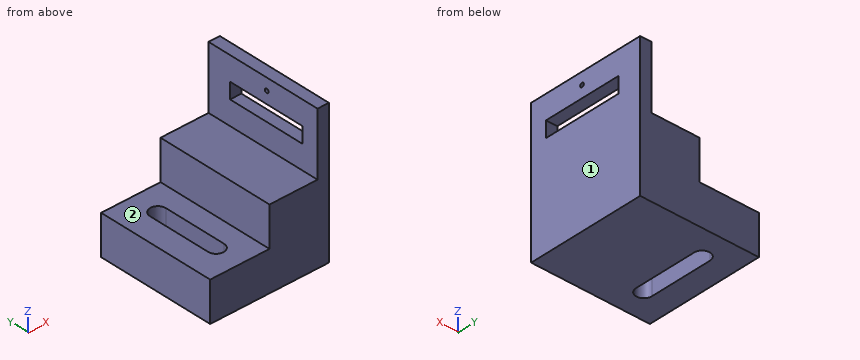
```python
from build123d import *

# Parameters (mm, degrees)
F1_DEPTH = 150
F3_DEPTH = 50.001
F4_W     = 100
F4_H     = 20
F4_R     = 2.5
F5_DEPTH = 14.313931


with BuildPart() as f1:
    # F0 (on Front) → F1 (new body)
    with BuildSketch(Plane.XZ):
        Polygon((-75, -90), (75, -90), (75, 90), (60.687069, 90), (60.687069, 10), (0, 10), (0, -40), (-75, -40), align=None)
    extrude(amount=F1_DEPTH)

    # F2 (on face) → F3 (cut, through all)
    with BuildSketch(Plane.XY.offset(-40)):
        with BuildLine():
            ThreePointArc((-45.374333, -35), (-35.374333, -45), (-25.374333, -35))
            ThreePointArc((-25.374333, -35), (-35.374333, -25), (-45.374333, -35))
        make_face()
        with BuildLine():
            Line((-25.374333, -115), (-25.374333, -35))
            ThreePointArc((-25.374333, -35), (-35.374333, -45), (-45.374333, -35))
            Line((-45.374333, -35), (-45.374333, -115))
            ThreePointArc((-45.374333, -115), (-35.374333, -105), (-25.374333, -115))
        make_face()
        with BuildLine():
            ThreePointArc((-45.374333, -115), (-35.374333, -125), (-25.374333, -115))
            ThreePointArc((-25.374333, -115), (-35.374333, -105), (-45.374333, -115))
        make_face()
    extrude(amount=-F3_DEPTH, mode=Mode.SUBTRACT)

    # F4 (on face) → F5 (cut, through all)
    with BuildSketch(Plane(origin=(60.687069, 0, 0), x_dir=(0, -1, 0), z_dir=(-1, 0, 0))):
        with Locations((79.612304, 50)):
            Rectangle(F4_W, F4_H)
        with Locations((80.003977, 75)):
            Circle(F4_R)
    extrude(amount=-F5_DEPTH, mode=Mode.SUBTRACT)


solid = f1.part
```
The listing builds one solid part. Answer for the finished solid, in the listing's coordinates (mm). Face numbers are marked on the shaded views. A direction names the side the tool comes from. Coordinates: 2 decimals unless noted, no trailing zeros. Write each loop counter-clockwise with the first axis right and the second up, starting at its lowest first coordinate (ties: lowest second). Pieces come first, ordered by that corner, then holes. Notation, with made-up numbers: M -26,32 L 18,32 A15 cw 18,59 Z; hole C 69,-8.75 d6. An arc over 180 degrees is marked long. Use a Markdown table: item, result. Add a question column.
1. Which of the six approach directions +Z, -Z, +X, -X, +Y, -Y give full straight-line access (tool end or side, diameter ignored) to the marked faces 1 and 2?
2. Given P1, Ø6.5, axis at y = -80, z = 75, coming from the -X side; P2, Ø8, axis at x = -2, y = -102.5, coming from the +Z side; P3, Ø25, axis at y = -107, z = -23.5, coming from the -X side, each flat-ended and moving along its own axis, determine where each tip first touches the part or whether it passes through.
3. Straight lines are drawn through the part: line 1 along Z through (x, y) = (25, -77.5); line 2 along X through (y, z) = (-78, 78.5); line 3 along Z through (x, y) = (-45, -133). For each, find the intervals that lie inside material, in ascending order. Write a range as [from, to].
4. Section B-B (z = -66) is taken. Give the vertices of the cut face in (x, y).
5. Section D-D (x = -37.5) is taken. Give the vertices of the cut face in (y, z).
6. Section A-A (y = -104) is taken. Give the vertices of the cut face in (x, z).
7. Section C-C (z = 75) is taken. Give the vertices of the cut face in (x, y), plus the area to 3 significant figures.
Data:
| question | item | result |
|---|---|---|
| 1 | face 1 | +Z, -Z, +X, +Y, -Y |
| 1 | face 2 | +Z, -X, +Y, -Y |
| 2 | P1 | stops at x = 60.69 |
| 2 | P2 | stops at z = 10 |
| 2 | P3 | stops at x = 0 |
| 3 | line 1 | z = [-90, 10] |
| 3 | line 2 | x = [60.69, 75] |
| 3 | line 3 | z = [-90, -40] |
| 4 | outline | M -75,-150 L 75,-150 L 75,0 L -75,0 Z; hole M -45.37,-115 A10 ccw -25.37,-115 L -25.37,-35 A10 ccw -45.37,-35 Z |
| 5 | outline | M -150,-90 L -124.77,-90 L -124.77,-40 L -150,-40 Z; M -25.23,-90 L 0,-90 L 0,-40 L -25.23,-40 Z |
| 6 | outline | M -75,-90 L -45.37,-90 L -45.37,-40 L -75,-40 Z; M -25.37,-90 L 75,-90 L 75,40 L 60.69,40 L 60.69,10 L 0,10 L 0,-40 L -25.37,-40 Z; M 60.69,60 L 75,60 L 75,90 L 60.69,90 Z |
| 7 | outline | M 60.69,-150 L 75,-150 L 75,-82.5 L 60.69,-82.5 Z; M 60.69,-77.5 L 75,-77.5 L 75,0 L 60.69,0 Z |
| 7 | area | 2,080 mm2 |
